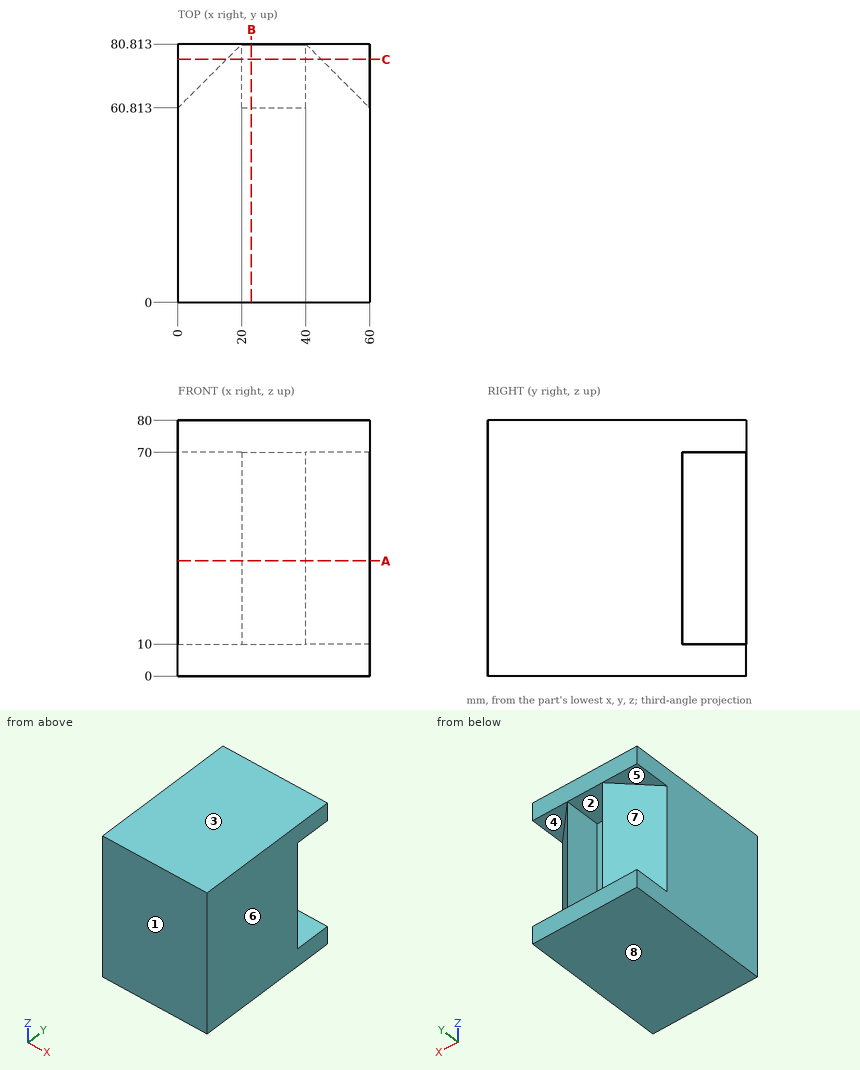
Part print with two shaded views. Sizes in mm from the minimum x, y, z corner. A direction names the side the tool comes from. Round coordinates to 2 decimals unless told otherwise and drop trailing zeros. Order: outer loops, then holes, each group sorted by start corner. A loop starts at its lowest first (then second) coordinate and runs counter-clockwise, first axis right, second up. Notation, with made-up numbers: (57.5, 45.5) -> (66.5, 45.5) arc R17 cw to (66.5, 57.5) -> close; hole circle Ø8 at (-25.75, 40). An arc over 180 degrees is marked (long way). Use one line per item in the form item = value.
Item 1: Tool access for the marked faces 1, 2, 3, 4 and 5: list every direction of +Z, -Z, +X, -X, +Y, -Y with a clear straight run to the whole face (end or side of a thin tool).
Returned:
face_1 = +Z, -Z, +X, -X, -Y
face_2 = +Y
face_3 = +Z, +X, -X, +Y, -Y
face_4 = +X, +Y
face_5 = -X, +Y
Item 2: Drill centre lines: line 1 (Y direction, x = 26, z = 66); line 2 (X direction, y = 63, z = 11.5) (1 decimal); line 3 (X direction, y = 63.5, z = 67) (1 decimal). Where is each one in solid material? Low to high.
Returned:
line_1 = 0 to 60.81
line_2 = 2.2 to 20, 40 to 57.8
line_3 = 2.7 to 20, 40 to 57.3
Item 3: Cut at A-A, the plane z = 36. Write the cut outline in (x, y), and give its area (3 significant figures).
Returned:
outline = (0, 0) -> (60, 0) -> (60, 60.81) -> (40, 80.81) -> (40, 60.81) -> (20, 60.81) -> (20, 80.81) -> (0, 60.81) -> close
area = 4,050 mm^2
Item 4: Cut at B-B, the plane x = 23. Write the cut outline in (y, z), and give its area (4 significant figures).
Returned:
outline = (0, 0) -> (80.81, 0) -> (80.81, 10) -> (60.81, 10) -> (60.81, 70) -> (80.81, 70) -> (80.81, 80) -> (0, 80) -> close
area = 5,265 mm^2
Item 5: Pull direction Z, two halves, no side cores. Call the marked faces 6, 7 and 8: released by +Z, released by -Z, zero draft, split by the parting line, or undercut.
Returned:
face_6 = zero draft
face_7 = undercut
face_8 = released by -Z
Item 6: Cut at C-C, the plane y = 76. Write the cut outline in (x, z), and give its area (3 significant figures).
Returned:
outline = (0, 0) -> (60, 0) -> (60, 10) -> (44.81, 10) -> (44.81, 70) -> (60, 70) -> (60, 80) -> (0, 80) -> (0, 70) -> (15.19, 70) -> (15.19, 10) -> (0, 10) -> close; hole (20, 10) -> (40, 10) -> (40, 70) -> (20, 70) -> close
area = 1,780 mm^2
Item 7: Flat gauge pins, fed straight in: pin 1 Ø10 at (x, z) = (27.5, 49) entering from +Y; pin 2 Ø6 at (y, z) = (71, 40.5) entering from -X; pin 3 Ø1.5 at (y, z) = (72, 60.5) entering from -X. Where does each tip first touch, or does it go through?
Returned:
pin_1 = 60.81
pin_2 = 7.19
pin_3 = 10.44
